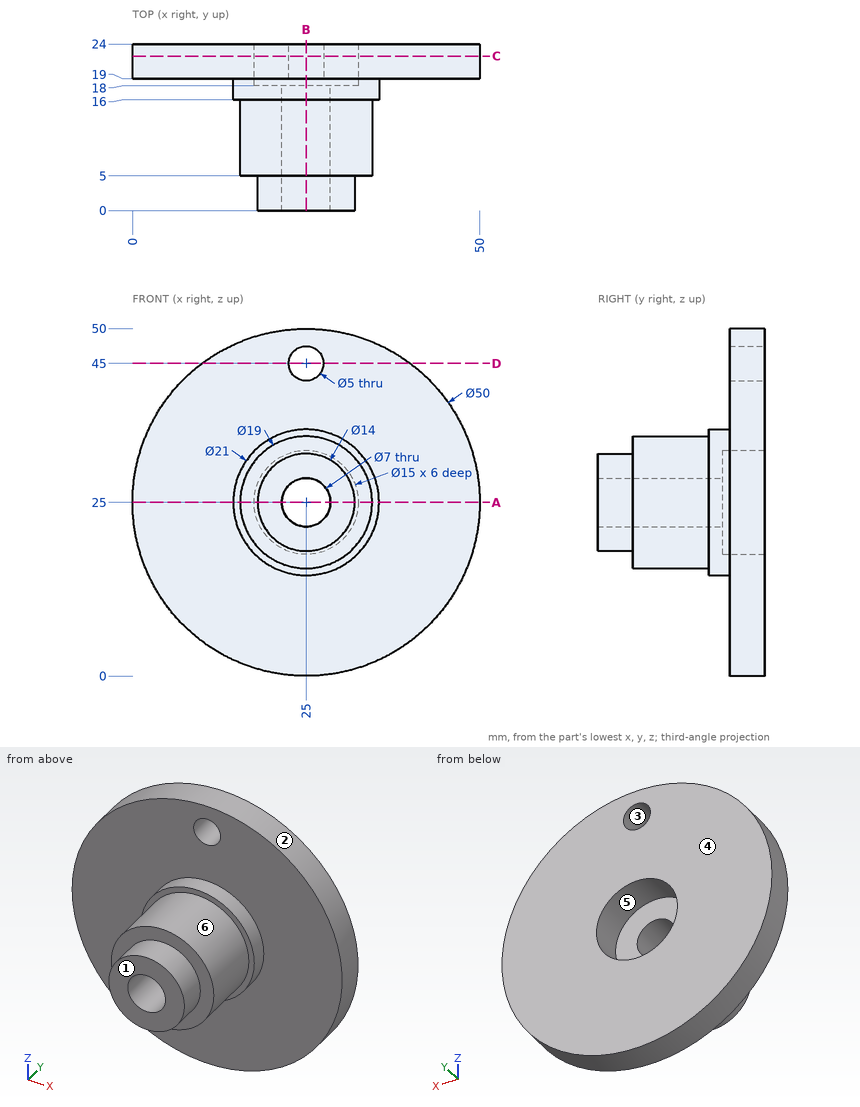
Source: three-view drawing plus pictorial views. Frame: mm from the lowest corner of the part. A direction names the side the tool comes from. Give positions to 0.01 mm unless a question says otherwise; leave off trailing zeros. Order: outer loops, then holes, each group sorted by start corner. A loop starts at its lowest first (then second) coordinate and runs counter-clockwise, first axis right, second up. Notation, with made-up numbers: (-13, 40.25) - (-9, 40.25) arc R7 cw to (-9, 50.25) - close; hole circle Ø3 at (-5.5, -27). An arc over 180 degrees is marked (long way). Put each result on its own line as item: value.
Item 1: Section query C-C, the plane y = 22.25. Return loops of the section in (x, z).
Found:
outline: circle Ø50 at (25, 25); hole circle Ø15 at (25, 25); hole circle Ø5 at (25, 45)
Item 2: Section query B-B, the plane x = 25. Return loops of the section in (y, z).
Found:
outline: (0, 18) - (5, 18) - (5, 15.5) - (16, 15.5) - (16, 14.5) - (19, 14.5) - (19, 0) - (24, 0) - (24, 17.5) - (18, 17.5) - (18, 21.5) - (0, 21.5) - close; (0, 28.5) - (18, 28.5) - (18, 32.5) - (24, 32.5) - (24, 42.5) - (19, 42.5) - (19, 35.5) - (16, 35.5) - (16, 34.5) - (5, 34.5) - (5, 32) - (0, 32) - close; (19, 47.5) - (24, 47.5) - (24, 50) - (19, 50) - close
Item 3: Access query for the marked faces 4, 5 and 6. Directions: +Z, -Z, +X, -X, +Y, -Y. A direction counts if a zero-diameter tool reaches every point of the face in a straight line with its end or side. Return the directions, or none.
Found:
face 4: +Z, -Z, +X, -X, +Y
face 5: +Y
face 6: -Y
Item 4: Section query D-D, the plane z = 45. Return loops of the section in (x, y), then the cut area to 3 significant figures.
Found:
outline: (10, 19) - (22.5, 19) - (22.5, 24) - (10, 24) - close; (27.5, 19) - (40, 19) - (40, 24) - (27.5, 24) - close
area: 125 mm^2
Item 5: Draft query along Z for the marked faces 1, 2 and 3. Return one class per face: +Z half, -Z half, draft (parallel to the pull), parting line (faces both ways), or undercut.
Found:
face 1: draft
face 2: parting line
face 3: undercut
Item 6: Contact query for flat-ended pins moving along their axis: pin 1 (10 mm diameter, centred on x = 15, y = 3.5, fed in from -Z); pin 2 (1.5 mm diameter, centred on x = 33, y = 5.5, fed in from -Z); pin 3 (13.5 mm diameter, centred on x = 25, z = 25, fed in from +Y). Output: stop coordinate, or through.
Found:
pin 1: stops at z = 17.07
pin 2: stops at z = 18.86
pin 3: stops at y = 18
Item 7: Section query A-A, the plane z = 25. Return loops of the section in (x, y), then the cut area to 3 significant figures.
Found:
outline: (0, 19) - (14.5, 19) - (14.5, 16) - (15.5, 16) - (15.5, 5) - (18, 5) - (18, 0) - (21.5, 0) - (21.5, 18) - (17.5, 18) - (17.5, 24) - (0, 24) - close; (28.5, 0) - (32, 0) - (32, 5) - (34.5, 5) - (34.5, 16) - (35.5, 16) - (35.5, 19) - (50, 19) - (50, 24) - (32.5, 24) - (32.5, 18) - (28.5, 18) - close
area: 376 mm^2
Item 8: Ray query, L1, parallel to Z at x = 25, y = 21.5; L2, parallel to Y at x = 32.5, z = 24; L3, parallel to Y at x = 34, z = 2. Return the intervals inside material, ascending. Write a range as from..to.
Found:
L1: z = 0..17.5, 32.5..42.5, 47.5..50
L2: y = 5..24
L3: y = 19..24
